Job drawing, mm, ordinate dimensions from the low corner. One solid piece. A direction names the side the tool comes from. Give positions to 0.01 mm unless a question says otherwise; leave off trailing zeros. Write each loop counter-clockwise with the first axis right and the second up, starting at its lowest first coordinate (ties: lowest second). Pieces come first, ordered by that corner, then holes. Notation, with made-up numbers: M 40,15.25 L 96,15.25 A30 cw 96,38.25 Z; hole C 45.25,49.25 d5. An arc over 180 degrees is marked long. Use CSV: the item, a comma, the result in double quotes. Start each with the question number.
Item 1: Cut at A-A (y = 16). List the corners of the cut face in (x, z) (1 decimal).
Item 2: Drill centre lines: line 1 (Y direction, x = 5, z = 4.5) (1 decimal); line 2 (X direction, y = 19, z = 3.25); line 3 (Z direction, x = 3.5, y = 2.5) (1 decimal). Where is each one in solid material? Low to high. Write a range as [from, to].
Item 3: Cut at B-B (y = 30). List the corners of the cut face in (x, z), then the cut area to 3 significant figures.
Item 4: Which spindle directions (+Z, -Z, +X, -X, +Y, -Y) get a long thin tool onto all of the face, cutting with end or side? Do the marked faces 1, 2 and 3. Say none if no direction does.
Item 5: Pin check, flat tips, straight feed: pin 1 (3 mm diameter, centred on x = 3, y = 3.5, fed in from +Z); pin 2 (2 mm diameter, centred on x = 1.5, z = 3, fed in from -Y). Stop position of each tip, or through.
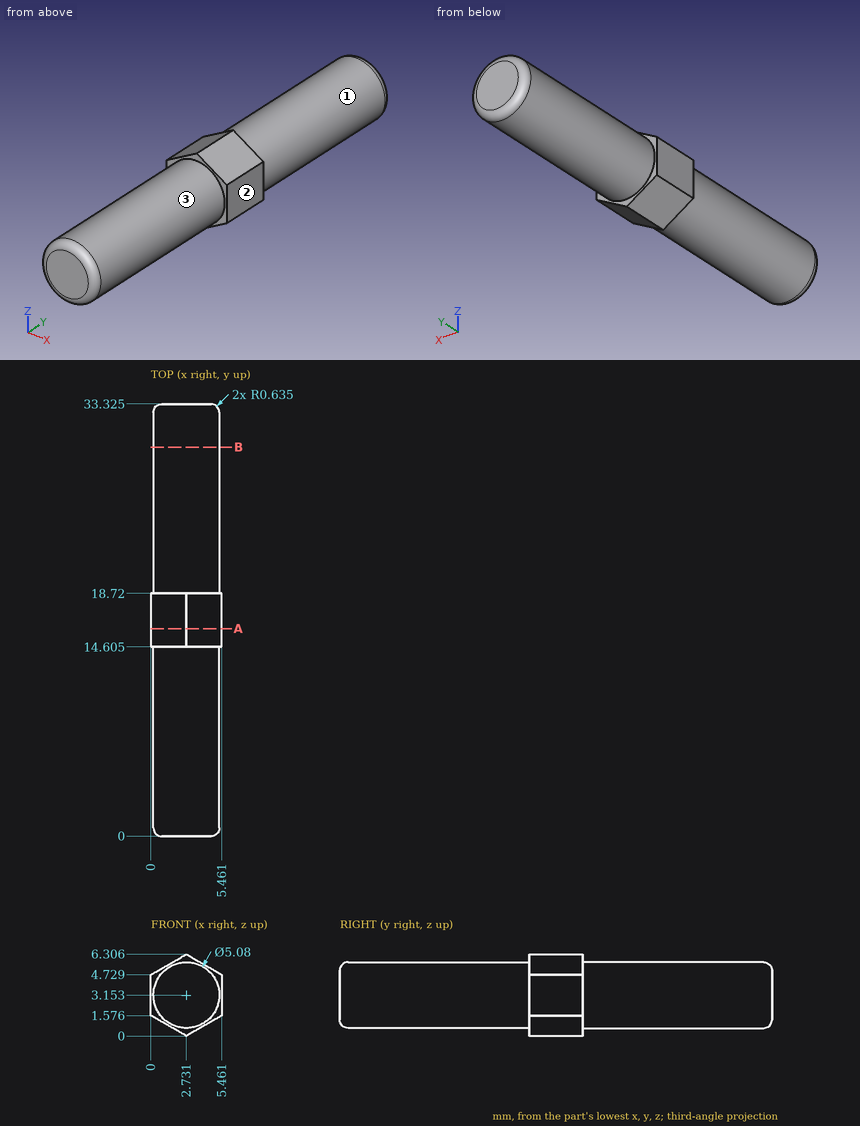
Worked answers:
1,outline,"M 0,1.6 L 2.7,0 L 5.5,1.6 L 5.5,4.7 L 2.7,6.3 L 0,4.7 Z"
2,line 1,"y = [14.6, 18.7]"
2,line 2,"x = [0.19, 5.27]"
2,line 3,"z = [0.7, 5.6]"
3,outline,"C 2.73,3.15 d5.08"
3,area,"20.3 mm^2"
4,face 1,"+Y"
4,face 2,"+Z, -Z, +X, +Y, -Y"
4,face 3,"-Y"
5,pin 1,"stops at z = 5.69"
5,pin 2,"stops at y = 0"
